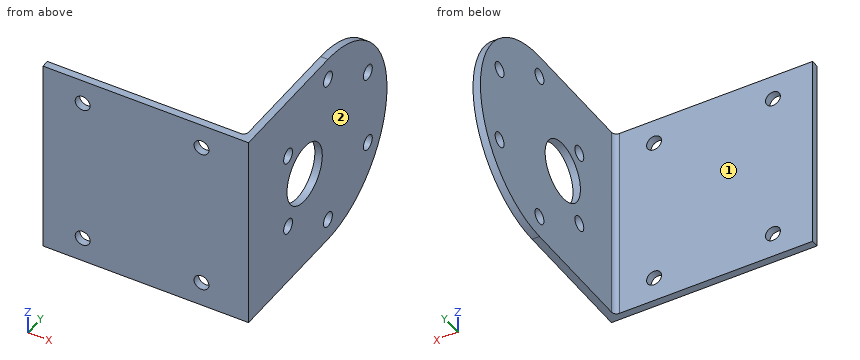
Autodesk Inventor part; units mm, degrees
ref_plane "YZ Plane" through (0, 0, 0) normal (1, 0, 0) x (0, 1, 0)
ref_plane "XZ Plane" through (0, 0, 0) normal (0, 1, 0) x (-1, 0, 0)
ref_plane "XY Plane" through (0, 0, 0) normal (0, 0, 1) x (1, 0, 0)
sketch "Sketch1" plane through (0, 0, 0) normal (0, 1, 0) x (-1, 0, 0)
  line L0 (-20, 20) -> (-20, -20)
  line L1 (-20, -20) -> (20, -20)
  line L2 (20, -20) -> (20, 20)
  line L3 (20, 20) -> (-20, 20)
  line L4 (-20, 20) -> (20, -20) construction
  line L5 (-20, -20) -> (20, 20) construction
  point P0 (0, 0)
  point P1 (0, -20)
  dimension "d0" = 40
  dimension "d1" = 40
extrude "Extrusion1" add sketch "Sketch1" along normal blind 1.5
sketch "Sketch2" plane through (20, 0, 20) normal (1, 0, 0) x (0, 0, -1)
  circle A0 centre (20, 26.9) radius 20
  line L0 (40, 1.5) -> (40, 46.9)
  line L1 (40, 1.5) -> (0, 1.5)
  line L2 (0, 1.5) -> (0, 46.9)
  line L3 (0, 46.9) -> (40, 46.9)
  line L4 (0, 0) -> (40, 0)
  line L5 (0, 0) -> (0, 1.5)
  line L6 (0, 1.5) -> (0, 0)
  line L7 (40, 0) -> (0, 0)
  line L8 (0, 0) -> (40, 0)
  line L9 (40, 0) -> (40, 1.5)
  line L10 (40, 0) -> (40, 1.5)
  point P0 (20, 0)
  point P1 (40, 26.9)
  point P2 (0, 26.9)
  dimension "d4" = 45.4
extrude "Extrusion2" add sketch "Sketch2" along normal blind 1.5 contours A0 | L0 L1 L2 A0 | L9 L4 L5 L1
fillet "Fillet1" radius 1 1 edges at (20, 1.5, 0)
sketch "Sketch3" plane through (21.5, 0, 20) normal (1, 0, 0) x (0, 0, -1)
  arc A0 (40, 26.9) -> (0, 26.9) centre (20, 26.9) ccw
  circle A1 centre (20, 26.9) radius 15.605
  circle A2 centre (20, 19) radius 5.98
  circle A3 centre (4.395, 26.9) radius 1.5
  point P0 (20, 0)
  dimension "d8" = 31.21
  dimension "d9" = 7.9
  dimension "d10" = 11.96
  dimension "d11" = 3
extrude "Extrusion3" cut sketch "Sketch3" against normal up to surface (1.5 mm away) contours A2
extrude "Extrusion4" cut sketch "Sketch3" against normal up to surface (1.5 mm away) contours A3 A1 | A1 A3 picked at (4.9003, 26.9) picked at (3.9042, 26.9621)
pattern_circular "Circular Pattern1" count 6 over 360 about axis through (20, 26.9, 0) along (1, 0, 0) of "Extrusion4"
sketch "Sketch4" plane through (0, 1.5, 0) normal (0, 1, 0) x (1, 0, 0)
  line L0 (12, 15) -> (-12, 15)
  line L1 (-12, 15) -> (-12, -15)
  line L2 (-12, -15) -> (12, -15)
  line L3 (12, -15) -> (12, 15)
  line L4 (-20, 20) -> (-20, -20)
  line L5 (-20, -20) -> (19, -20)
  circle A0 centre (-12, 15) radius 1.5
  point P0 (0, 0)
  dimension "d19" = 30
  dimension "d20" = 24
  dimension "d21" = 8
  dimension "d22" = 5
  dimension "d23" = 3
extrude "Extrusion5" cut sketch "Sketch4" against normal up to surface (1.5 mm away) contours A0 L1 L0 | L0 L1 A0
pattern_linear "Rectangular Pattern1" count 2 spacing 24 along (1, 0, 0) count 2 spacing 30 along (0, 0, 1) of "Extrusion5"
properties part number "motor_support"
Verification items for the finished model (mm, model axes). Face numbers are marked on the shaded views. A direction names the side the tool comes from. Coordinates: 2 decimals unless noted, no trailing zeros. Write each loop counter-clockwise with the first axis right and the second up, starting at its lowest first coordinate (ties: lowest second). Pieces come first, ordered by that corner, then holes. Notation, with made-up numbers: (48, -6.75) - (93, -6.75) arc R34 ccw to (93, 31.25) - close; hole circle Ø10 at (49.5, 60). An arc over 180 degrees is marked (long way). Write item = value, one per line.
Q1. Cross-section at C-C (y = 21.5). Enter the section's corners in (x, z).
Answer:
outline = (20, -20) - (21.5, -20) - (21.5, -5.43) - (20, -5.43) - close; (20, 5.43) - (21.5, 5.43) - (21.5, 20) - (20, 20) - close
Q2. Cross-section at B-B (x = -12). Enter the section's corners in (y, z), plus the area to 3 significant figures.
Answer:
outline = (0, -20) - (1.5, -20) - (1.5, -16.5) - (0, -16.5) - close; (0, -13.5) - (1.5, -13.5) - (1.5, 13.5) - (0, 13.5) - close; (0, 16.5) - (1.5, 16.5) - (1.5, 20) - (0, 20) - close
area = 51.0 mm²
Q3. Access from +Z, -Z, +X, -X, +Y, -Y to the whole of each face (thin tool, end or side, straight path). Record for the marked faces 1 and 2.
Answer:
face_1 = +Z, -Z, -X, +Y
face_2 = +Z, -Z, +X, +Y, -Y
Q4. Go/stop test with flat-tipped pins: pin 1 Ø4 at (y, z) = (26.9, -15.605) entering from -X; pin 2 Ø2.5 at (x, z) = (-12, -15) entering from -Y; pin 3 Ø12 at (x, z) = (4, 0) entering from +Y. Record where each tip stops, or that it passes through.
Answer:
pin_1 = 20
pin_2 = through
pin_3 = 1.5
Q5. Cross-section at A-A (z = 0). Enter the section's corners in (x, y).
Answer:
outline = (-20, 0) - (21.5, 0) - (21.5, 13.02) - (20, 13.02) - (20, 2.5) arc R1 cw to (19, 1.5) - (-20, 1.5) - close; (20, 24.98) - (21.5, 24.98) - (21.5, 46.9) - (20, 46.9) - close
Q6. Cross-section at D-D (z = 8.5). Enter the section's corners in (x, y).
Answer:
outline = (-20, 0) - (21.5, 0) - (21.5, 12.06) - (20, 12.06) - (20, 2.5) arc R1 cw to (19, 1.5) - (-20, 1.5) - close; (20, 14.71) - (21.5, 14.71) - (21.5, 39.09) - (20, 39.09) - close; (20, 41.74) - (21.5, 41.74) - (21.5, 45) - (20, 45) - close
Q7. Material ranges on L1, parallel to Z at x = -12, y = 1.15; L2, parallel to X at y = 23.5, z = -9; L3, parallel to Y at x = -3, z = 13, recorded low to high. Write a range as from..to.
Answer:
L1 = -20..-16.5, -13.5..13.5, 16.5..20
L2 = 20..21.5
L3 = 0..1.5
